Could you check a few things on this model? Use its own coordinates, in mm. Face numbers are marked on the shaded views. A direction names the side the tool comes from. Round coordinates to 2 decimals unless told otherwise and drop trailing zeros. Loops run counter-clockwise (first coordinate to the right, second up) from the corner with the lowest first, then second, coordinate; pieces in that order, holes last.
from build123d import *

# Parameters (mm, degrees)
SKETCH1_R           = 31.75
BOSS_EXTRUDE1_DEPTH = 12.7
SKETCH2_R           = 4.7625
CUT_EXTRUDE1_DEPTH  = 25.4
CIRPATTERN1_COUNT   = 3


with BuildPart() as part:
    # Sketch1 → Boss-Extrude1 (new, symmetric)
    with BuildSketch(Plane.XY):
        with BuildLine():
            Line((-51.195336702, 0), (-51.195336702, 102.193578565))
            Line((-51.195336702, 102.193578565), (-6.35, 102.193578565))
            Line((-6.35, 102.193578565), (-6.35, 50.8))
            Line((-6.35, 50.8), (6.35, 50.8))
            ThreePointArc((6.35, 50.8), (16.297475531, 48.531997603), (25.597668351, 44.336462139))
            Line((25.597668351, 44.336462139), (114.099903492, -6.760327144))
            Line((114.099903492, -6.760327144), (91.677235141, -45.597527969))
            Line((91.677235141, -45.597527969), (47.169090512, -19.900738686))
            Line((47.169090512, -19.900738686), (40.819090512, -30.899261314))
            ThreePointArc((40.819090512, -30.899261314), (33.881205055, -38.380026629), (25.597668351, -44.336462139))
            Line((25.597668351, -44.336462139), (-62.90456679, -95.433251422))
            Line((-62.90456679, -95.433251422), (-85.327235141, -56.596050597))
            Line((-85.327235141, -56.596050597), (-40.819090512, -30.899261314))
            Line((-40.819090512, -30.899261314), (-47.169090512, -19.900738686))
            ThreePointArc((-47.169090512, -19.900738686), (-50.178680586, -10.151970974), (-51.195336702, 0))
        make_face()
        Circle(SKETCH1_R, mode=Mode.SUBTRACT)
    extrude(amount=BOSS_EXTRUDE1_DEPTH, both=True)

    # Sketch2 → Cut-Extrude1 (cut)
    with BuildSketch(Plane(origin=(-6.35, 0, 0), x_dir=(0, 0, -1), z_dir=(1, 0, 0))):
        with Locations(Location((0, 76.2, 0), (0, 0, 90))):
            Circle(SKETCH2_R)
    cut_extrude1 = extrude(amount=-CUT_EXTRUDE1_DEPTH, mode=Mode.SUBTRACT)

    # CirPattern1: Cut-Extrude1 ×3 about axis
    cirpattern1_axis = Axis((0, 0, 0), (0, 0, 1))
    for i in range(1, CIRPATTERN1_COUNT):
        add(cut_extrude1.rotate(cirpattern1_axis, i * 360 / CIRPATTERN1_COUNT), mode=Mode.SUBTRACT)


solid = part.part
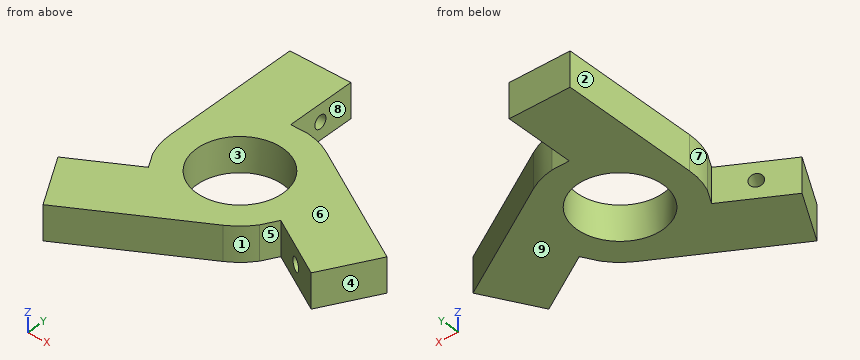
Item 1: Will these pins go through, and if not, where does the flat tip stop? pin 1 (8 mm diameter, centred on x = 20, z = -4, fed in from -Y); pin 2 (2 mm diameter, centred on y = 71.5, z = 9, fed in from +X); pin 3 (3 mm diameter, centred on y = 76, z = -1.5, fed in from +X).
Results list:
pin 1: stops at y = -49.88
pin 2: stops at x = -6.35
pin 3: stops at x = -31.75
Item 2: If we section it at A-A, the plane y = 76.2: Please give me the cut outline in (x, z), then the cut area to 3 significant figures.
Results list:
outline: (-51.2, -12.7) - (-6.35, -12.7) - (-6.35, -4.76) - (-31.75, -4.76) - (-31.75, 4.76) - (-6.35, 4.76) - (-6.35, 12.7) - (-51.2, 12.7) - close
area: 897 mm2
Item 3: If we section it at B-B, the plane x = 19.5: Please give me the cut outline in (y, z), then the cut area to 3 significant figures.
Results list:
outline: (-47.86, -12.7) - (-25.06, -12.7) - (-25.06, 12.7) - (-47.86, 12.7) - close; (25.06, -12.7) - (47.34, -12.7) - (47.34, 12.7) - (25.06, 12.7) - close
area: 1,150 mm2
Item 4: We'd pull the mould along X, two halves only. Please class the marked faces 1, 2, 3 and 4: released by +X, released by -X, zero draft, split by the parting line, or undercut.
Results list:
face 1: undercut
face 2: released by -X
face 3: undercut
face 4: released by +X
Item 5: If we section it at C-C, the plane x = -22.5: Please give me the cut outline in (y, z) (1 decimal).
Results list:
outline: (-72.1, -12.7) - (-22.4, -12.7) - (-22.4, 12.7) - (-72.1, 12.7) - close; (22.4, -12.7) - (102.2, -12.7) - (102.2, 12.7) - (22.4, 12.7) - close; hole circle Ø9.5 at (76.2, 0)
Item 6: If we section it at D-D, the plane z = 0: Please give me the cut outline in (x, y), then the cut area to 3 significant figures.
Results list:
outline: (-85.33, -56.6) - (-62.9, -95.43) - (25.6, -44.34) arc R51.2 ccw to (40.82, -30.9) - (47.17, -19.9) - (65.04, -30.22) - (77.74, -8.22) - (85.99, -12.98) - (73.29, -34.98) - (91.68, -45.6) - (114.1, -6.76) - (25.6, 44.34) arc R51.2 ccw to (6.35, 50.8) - (-6.35, 50.8) - (-6.35, 71.44) - (-31.75, 71.44) - (-31.75, 80.96) - (-6.35, 80.96) - (-6.35, 102.19) - (-51.2, 102.19) - (-51.2, 0) arc R51.2 ccw to (-47.17, -19.9) - (-40.82, -30.9) - (-58.69, -41.22) - (-45.99, -63.22) - (-54.24, -67.98) - (-66.94, -45.98) - close; hole circle Ø63.5 at (0, 0)
area: 12,900 mm2
Item 7: For the marked faces 5, 6, 7, 8 and 9, which set-ups out of +Z, -Z, +X, -X, +Y, -Y let a thin tool reach every point of the face, with its end or its side?
Results list:
face 5: +Z, -Z, -Y
face 6: +Z, +X, -X, +Y, -Y
face 7: +Z, -Z, -X
face 8: +Z, -Z, +X, +Y
face 9: -Z, +X, -X, +Y, -Y
Item 8: If I drill on line 1 along Z through (x, y) = (-24, 76); line 2 along Y through (x, z) = (-21, 3.5); line 3 along Y through (x, z) = (0, -0.75), over which ranges is the centre line in solid material (lowest first)?
Results list:
line 1: z = -12.7 to -4.76, 4.76 to 12.7
line 2: y = -71.24 to -23.81, 23.81 to 72.97, 79.43 to 102.19
line 3: y = -59.12 to -31.75, 31.75 to 50.8
